Check sheet for the modelled part. Datum: model origin and axes. Units: mm. A direction names the side the tool comes from. Coordinates: 2 decimals unless noted, no trailing zeros. Loops run counter-clockwise (first coordinate to the right, second up) from the corner with the lowest first, then second, coordinate; pieces in that order, holes last.
```python
from build123d import *

# Parameters (mm, degrees)
EXTRUDE_3_DEPTH                 = 5
HOLE_WIZARD_M3_1_D              = 2.5
HOLE_WIZARD_M3_1_CSINK_D        = 3.05
HOLE_WIZARD_M3_1_CSINK_ANGLE    = 90
HOLE_WIZARD_M3_2_D              = 2.5
HOLE_WIZARD_M3_2_CSINK_D        = 3.05
HOLE_WIZARD_M3_2_CSINK_ANGLE    = 90
HOLE_WIZARD_6_0_6_1_D           = 6
HOLE_WIZARD_6_0_6_1_CSINK_D     = 6.05
HOLE_WIZARD_6_0_6_1_CSINK_ANGLE = 90
SKETCH_20_R                     = 2.4
CUT_EXTRUDE_2_DEPTH             = 192.006108105
HOLE_WIZARD_M6_2_D              = 5
HOLE_WIZARD_M6_2_CSINK_D        = 6.05
HOLE_WIZARD_M6_2_CSINK_ANGLE    = 90
EXTRUDE_5_DEPTH                 = 5
HOLE_WIZARD_M6_3_D              = 5
HOLE_WIZARD_M6_3_CSINK_D        = 6.05
HOLE_WIZARD_M6_3_CSINK_ANGLE    = 90


with BuildPart() as part:
    # 草图8 → 凸台-拉伸3 (new body)
    with BuildSketch(Plane.XY):
        Polygon((144.337567297, 0), (72.168783649, 125), (-72.168783649, 125), (-144.337567297, 0), (-72.168783649, -125), (-40, -125), (-40, -95), (40, -95), (40, -125), (72.168783649, -125), align=None)
    extrude(amount=EXTRUDE_3_DEPTH)

    # M3 螺纹孔1 (through all)
    with Locations(Plane.XY.offset(5)):
        with Locations((-30, -85)):
            hole_wizard_m3_1 = CounterSinkHole(HOLE_WIZARD_M3_1_D / 2, HOLE_WIZARD_M3_1_CSINK_D / 2, counter_sink_angle=HOLE_WIZARD_M3_1_CSINK_ANGLE)

    # M3 螺纹孔2 (through all)
    with Locations(Plane.XY.offset(5)):
        with Locations((-30, 89.511250681)):
            hole_wizard_m3_2 = CounterSinkHole(HOLE_WIZARD_M3_2_D / 2, HOLE_WIZARD_M3_2_CSINK_D / 2, counter_sink_angle=HOLE_WIZARD_M3_2_CSINK_ANGLE)

    # 镜向1: M3 螺纹孔1, M3 螺纹孔2 across plane
    add(hole_wizard_m3_1.mirror(Plane(origin=(0, 0, 0), x_dir=(0, 0, 1), z_dir=(1, 0, 0))), mode=Mode.SUBTRACT)
    add(hole_wizard_m3_2.mirror(Plane(origin=(0, 0, 0), x_dir=(0, 0, 1), z_dir=(1, 0, 0))), mode=Mode.SUBTRACT)

    # Ø6.0 (6) 直径孔1 (through all)
    with Locations(Plane.XY.offset(5)):
        with Locations((-135.003092598, 0), (-67.980688817, -118.866778441), (-67.980688817, 117.662022204)):
            hole_wizard_6_0_6_1 = CounterSinkHole(HOLE_WIZARD_6_0_6_1_D / 2, HOLE_WIZARD_6_0_6_1_CSINK_D / 2, counter_sink_angle=HOLE_WIZARD_6_0_6_1_CSINK_ANGLE)

    # 镜向2: Ø6.0 (6) 直径孔1 across plane
    add(hole_wizard_6_0_6_1.mirror(Plane(origin=(0, 0, 0), x_dir=(0, 0, 1), z_dir=(1, 0, 0))), mode=Mode.SUBTRACT)

    # 草图20 → 切除-拉伸2 (cut, through all)
    with BuildSketch(Plane.XY.offset(5)):
        with Locations((56.370867728, 13.653021969)):
            Circle(SKETCH_20_R)
        with Locations((105.370867728, 13.324633606)):
            Circle(SKETCH_20_R)
        with Locations((56.370867728, -14.346978031)):
            Circle(SKETCH_20_R)
        with Locations((105.370867728, -14.346978031)):
            Circle(SKETCH_20_R)
    extrude(amount=-CUT_EXTRUDE_2_DEPTH, mode=Mode.SUBTRACT)

    # M6 螺纹孔2 (through all)
    with Locations(Plane.XY.offset(5)):
        with Locations((-121.691346762, -29.681796734), (122.33153109, -29.681796734), (-121.691346762, 29.648282418), (122.33153109, 29.648282418)):
            CounterSinkHole(HOLE_WIZARD_M6_2_D / 2, HOLE_WIZARD_M6_2_CSINK_D / 2, counter_sink_angle=HOLE_WIZARD_M6_2_CSINK_ANGLE)

    # 草图28 → 凸台-拉伸5 (add)
    with BuildSketch(Plane.XY):
        Polygon((192.254989682, -41.465529773), (96.127494841, 125.032175296), (-96.127494841, 125.032175296), (-192.254989682, -41.465529773), (-96.127494841, -207.963234842), (96.127494841, -207.963234842), align=None)
    extrude(amount=-EXTRUDE_5_DEPTH)

    # M6 螺纹孔3 (through all)
    with Locations(Plane.XY.offset(5)):
        with Locations((-121.691346762, 29.648282418), (-135.003092598, 0), (-121.691346762, -29.681796734), (122.33153109, 29.648282418), (135.003092598, 0), (122.33153109, -29.681796734), (67.980688817, -118.866778441), (-67.980688817, -118.866778441), (67.980688817, 117.662022204), (-67.980688817, 117.662022204)):
            CounterSinkHole(HOLE_WIZARD_M6_3_D / 2, HOLE_WIZARD_M6_3_CSINK_D / 2, counter_sink_angle=HOLE_WIZARD_M6_3_CSINK_ANGLE)


solid = part.part
```
1) Section check B-B on z = 2.75. Give the number of separate pieces and of enclosed holes in the cut face, plus the area to 3 significant figures.
Answer sheet:
separate pieces: 1
enclosed holes: 18
area: 51,400 mm2
2) Section check C-C on y = -147.5. Enter the section's corners in (x, z).
Answer sheet:
outline: (-131.04, -5) - (131.04, -5) - (131.04, 0) - (-131.04, 0) - close
3) Set-up check for faces 1 (the flat face through (-107.75, 63.37, 2.46)), 2 (the flat face through (-1, -115, 0)), 3 (the flat face through (108.758, 61.625, 2.465)), 4 (the flat face through (-108.758, -61.625, 2.465)): record each of +Z, -Z, +X, -X, +Y, -Y from which the full face is reachable in a straight line by a thin tool's end or side.
Answer sheet:
face 1: +Z, -X, +Y
face 2: +Z
face 3: +Z, +X, +Y
face 4: +Z, -X, -Y
4) Scan lines: line 1 (Y direction, x = -30, z = 2.65); line 2 (Y direction, x = 122, z = 2.5); line 3 (X direction, y = -31.5, z = -1.25). Record each from-to range of solid material in increasing order.
Answer sheet:
line 1: y = -95 to -86.25, -83.75 to 88.26, 90.76 to 125
line 2: y = -38.69 to -32.16, -27.2 to 27.17, 32.13 to 38.69
line 3: x = -186.5 to -123.41, -119.98 to 120.62, 124.05 to 186.5
5) Depth check by flat-ended pin: pin 1 (1.8 mm diameter, centred on x = 68.5, y = 117.5, fed in from +Z); pin 2 (6 mm diameter, centred on x = -113, y = -155.5, fed in from +Z); pin 3 (1.2 mm diameter, centred on x = -29.5, y = -85.5, fed in from +Z); pin 4 (4 mm diameter, centred on y = -106.5, z = 3.5, fed in from -X). Enter the tip coordinate at first touch or a pass-through.
Answer sheet:
pin 1: passes through
pin 2: stops at z = 0
pin 3: stops at z = 4.78
pin 4: stops at x = -84
